For this review, take the finished solid that the model builds, in its own axes (mm). A direction names the side the tool comes from. Give positions to 0.01 mm unless a question says otherwise; leave off trailing zeros. Loops run counter-clockwise (first coordinate to the right, second up) from the corner with the lowest first, then second, coordinate; pieces in that order, holes last.
```python
from build123d import *

# Parameters (mm, degrees)
SKETCH1_R               = 400
BOSS_EXTRUDE1_DEPTH     = 50
SKETCH2_W               = 21
SKETCH2_H               = 21
BOSS_EXTRUDE2_DEPTH     = 20
SKETCH4_W               = 18.5
SKETCH4_H               = 21
CUT_EXTRUDE1_DEPTH      = 20
CUT_EXTRUDE2_DEPTH      = 793.881453939
CUT_EXTRUDE2_DEPTH_BACK = 793.881453939
SKETCH5_R               = 2
SKETCH6_R               = 4.380137325
SKETCH6_R_2             = 5.425166138
SKETCH6_R_3             = 8.421376202
SKETCH6_R_4             = 2.814926411
SKETCH6_R_5             = 5.941885297
SKETCH6_R_6             = 3.197207439
SKETCH6_R_7             = 2.027882418
CUT_EXTRUDE3_DEPTH      = 10


with BuildPart() as part:
    # Sketch1 → Boss-Extrude1 (new body)
    with BuildSketch(Plane.XY):
        Circle(SKETCH1_R)
    extrude(amount=BOSS_EXTRUDE1_DEPTH)

    # Sketch2 → Boss-Extrude2 (add)
    with BuildSketch(Plane.XY.offset(50)):
        with Locations((339.5, -60.5)):
            Rectangle(SKETCH2_W, SKETCH2_H)
        with Locations((339.5, 60.5)):
            Rectangle(SKETCH2_W, SKETCH2_H)
        with Locations((270.5, -170.5)):
            Rectangle(SKETCH2_W, SKETCH2_H)
        with Locations((270.5, 170.5)):
            Rectangle(SKETCH2_W, SKETCH2_H)
        with Locations((-270.5, -170.5)):
            Rectangle(SKETCH2_W, SKETCH2_H)
        with Locations((-339.5, -60.5)):
            Rectangle(SKETCH2_W, SKETCH2_H)
        with Locations((-339.5, 60.5)):
            Rectangle(SKETCH2_W, SKETCH2_H)
        with Locations((-270.5, 170.5)):
            Rectangle(SKETCH2_W, SKETCH2_H)
    extrude(amount=BOSS_EXTRUDE2_DEPTH)

    # Sketch4 → Cut-Extrude1 (cut)
    with BuildSketch(Plane.XY.offset(70)):
        with Locations((270.5, 170.5)):
            Rectangle(SKETCH4_W, SKETCH4_H)
        with Locations((339.5, 60.5)):
            Rectangle(SKETCH4_W, SKETCH4_H)
        with Locations((339.5, -60.5)):
            Rectangle(SKETCH4_W, SKETCH4_H)
        with Locations((270.5, -170.5)):
            Rectangle(SKETCH4_W, SKETCH4_H)
        with Locations((-270.5, -170.5)):
            Rectangle(SKETCH4_W, SKETCH4_H)
        with Locations((-339.5, -60.5)):
            Rectangle(SKETCH4_W, SKETCH4_H)
        with Locations((-339.5, 60.5)):
            Rectangle(SKETCH4_W, SKETCH4_H)
        with Locations((-270.5, 170.5)):
            Rectangle(SKETCH4_W, SKETCH4_H)
    extrude(amount=-CUT_EXTRUDE1_DEPTH, mode=Mode.SUBTRACT)

    # Sketch5 → Cut-Extrude2 (cut, two sides: drawn at the far end of the back side and taken through both)
    with BuildSketch(Plane(origin=(281, 0, 0), x_dir=(0, 0, -1), z_dir=(1, 0, 0)).offset(-CUT_EXTRUDE2_DEPTH_BACK)):
        with Locations((-62, 170.5)):
            Circle(SKETCH5_R)
        with Locations((-62, 60.5)):
            Circle(SKETCH5_R)
        with Locations((-62, -60.5)):
            Circle(SKETCH5_R)
        with Locations((-62, -170.5)):
            Circle(SKETCH5_R)
    extrude(amount=CUT_EXTRUDE2_DEPTH + CUT_EXTRUDE2_DEPTH_BACK, mode=Mode.SUBTRACT)

    # Sketch6 → Cut-Extrude3 (cut)
    with BuildSketch(Plane(origin=(0, 0, 0), x_dir=(-1, 0, 0), z_dir=(0, 0, -1))):
        with Locations((298.667764573, -172.435914274)):
            Circle(SKETCH6_R)
        with Locations((0, 342.463612446)):
            Circle(SKETCH6_R_2)
        with Locations((-298.667764573, -172.435914274)):
            Circle(SKETCH6_R_3)
        with Locations((276.746350043, -159.779579694)):
            Circle(SKETCH6_R_4)
        with Locations((-276.746350043, -159.779579694)):
            Circle(SKETCH6_R_5)
        with Locations((0, 311.235670646)):
            Circle(SKETCH6_R_6)
        with Locations((263.641581449, -152.213538019)):
            Circle(SKETCH6_R_7)
    extrude(amount=-CUT_EXTRUDE3_DEPTH, mode=Mode.SUBTRACT)


solid = part.part
```
Item 1: Take a section at C-C on x = 72. Give the boundary of the cut face in (y, z).
Answer:
outline: (-393.47, 0) - (393.47, 0) - (393.47, 50) - (-393.47, 50) - close
Item 2: Take a section at B-B on y = 0. Give the boundary of the cut face in (x, z), and give its area (3 significant figures).
Answer:
outline: (-400, 0) - (400, 0) - (400, 50) - (-400, 50) - close
area: 40,000 mm2
Item 3: For L1, parallel to Y at x = 280.05, z = 62; L2, parallel to Z at x = 329.4, y = 60.5; L3, parallel to Z at x = -189, y = 274.5, list the stretches that pass through material, from the lowest coordinate up.
Answer:
L1: y = -181 to -172.5, -168.5 to -160, 160 to 168.5, 172.5 to 181
L2: z = 0 to 60, 64 to 70
L3: z = 0 to 50
Item 4: Clearance check with flat-ended pins moving along their axes: pin 1 Ø6 at (x, y) = (-121.5, 253) entering from -Z; pin 2 Ø2 at (y, z) = (250.5, 31) entering from +X; pin 3 Ø5 at (x, y) = (302.5, -171.5) entering from -Z; pin 4 Ø12 at (x, z) = (101, 14.5) entering from +Y (3 decimals). State where each tip first meets the part, or that it passes through.
Answer:
pin 1: stops at z = 0
pin 2: stops at x = 312.65
pin 3: stops at z = 10
pin 4: stops at y = 388.555
Item 5: Tool access review of faces 5 (the flat face through (-348.75, -61, 58)), 6 (the flat face through (281, 170, 58)), 7 (the flat face through (-350, 60, 58)): name each direction out of +Z, -Z, +X, -X, +Y, -Y from which nothing blocks a thin tool from reaching the whole face with its end or side.
Answer:
face 5: +Z, +Y, -Y
face 6: +Z, +X, +Y, -Y
face 7: +Z, -X, +Y, -Y
Item 6: Take a section at A-A on z = 29. Give the boundary of the cut face in (x, y), and give its area (3 significant figures).
Answer:
outline: circle Ø800 at (0, 0)
area: 503,000 mm2
Item 7: The part is to be moulded in two halves that separate along X. For faces 1 (the flat face through (348.75, -61, 58)), 2 (the cylindrical face through (381.53, 120.15, 24.65)), 3 (the flat face through (-350, -61, 58)), 4 (the flat face through (261.25, -171, 58)), say which applies: released by +X, released by -X, zero draft, split by the parting line, or undercut.
Answer:
face 1: undercut
face 2: split by the parting line
face 3: released by -X
face 4: undercut
